Input: part model. Units: mm. Frame: model coordinates. A direction names the side the tool comes from. Coordinates: 2 decimals unless noted, no trailing zeros. Write each loop counter-clockwise with the first axis right and the second up, starting at its lowest first coordinate (ties: lowest second). Pieces come first, ordered by that corner, then holes. Notation, with made-up numbers: M -23,52 L 23,52 A16 ccw 23,72 Z; hole C -28.75,43.5 d3. An arc over 180 degrees is marked long. Use one line per item in the form item = value.
from build123d import *

# Parameters (mm, degrees)
SKETCH1_W                                       = 38.5
SKETCH1_H                                       = 70.536099416
BOSS_EXTRUDE1_DEPTH                             = 38
BOSS_EXTRUDE2_DEPTH                             = 4
BOSS_EXTRUDE3_START                             = -70.536099
BOSS_EXTRUDE3_DEPTH                             = 4
SKETCH4_W                                       = 62.536099416
SKETCH4_H                                       = 60
SKETCH4_R                                       = 17
SKETCH4_R_2                                     = 2.5
BOSS_EXTRUDE4_DEPTH                             = 2
CSK_FOR_M6_FLAT_HEAD_MACHINE_SCREW1_D           = 6.6
CSK_FOR_M6_FLAT_HEAD_MACHINE_SCREW1_CSINK_D     = 12.6
CSK_FOR_M6_FLAT_HEAD_MACHINE_SCREW1_CSINK_ANGLE = 90


with BuildPart() as part:
    # Sketch1 → Boss-Extrude1 (new body)
    with BuildSketch(Plane(origin=(0, 0, 502.500831462), x_dir=(1, 0, 0), z_dir=(0, 0, -1))):
        with Locations((165.241839146, 0)):
            Rectangle(SKETCH1_W, SKETCH1_H)
    extrude(amount=BOSS_EXTRUDE1_DEPTH)

    # Sketch3 → Boss-Extrude2 (add)
    with BuildSketch(Plane(origin=(0, 35.268049708, 0), x_dir=(-1, 0, 0), z_dir=(0, 1, 0))):
        Polygon((-184.491839146, 404.500831462), (-179.491839146, 404.500831462), (-145.991839146, 464.500831462), (-184.491839146, 464.500831462), align=None)
    extrude(amount=-BOSS_EXTRUDE2_DEPTH)

    # Sketch3<2> → Boss-Extrude3 (add)
    with BuildSketch(Plane(origin=(0, 35.268049708, 0), x_dir=(-1, 0, 0), z_dir=(0, 1, 0)).offset(BOSS_EXTRUDE3_START)):
        Polygon((-184.491839146, 404.500831462), (-179.491839146, 404.500831462), (-145.991839146, 464.500831462), (-184.491839146, 464.500831462), align=None)
    extrude(amount=BOSS_EXTRUDE3_DEPTH)

    # Sketch4 → Boss-Extrude4 (add)
    with BuildSketch(Plane.YZ.offset(184.491839146)):
        with Locations((0, 434.500831462)):
            Rectangle(SKETCH4_W, SKETCH4_H)
        with Locations(Location((0, 424.500831462, 0), (0, 0, 270))):
            Circle(SKETCH4_R, mode=Mode.SUBTRACT)
        with Locations(Location((-24.75, 459.250831462, 0), (0, 0, 270))):
            Circle(SKETCH4_R_2, mode=Mode.SUBTRACT)
        with Locations(Location((24.75, 459.250831462, 0), (0, 0, 270))):
            Circle(SKETCH4_R_2, mode=Mode.SUBTRACT)
        with Locations(Location((24.75, 409.750831462, 0), (0, 0, 270))):
            Circle(SKETCH4_R_2, mode=Mode.SUBTRACT)
        with Locations(Location((-24.75, 409.750831462, 0), (0, 0, 270))):
            Circle(SKETCH4_R_2, mode=Mode.SUBTRACT)
    extrude(amount=-BOSS_EXTRUDE4_DEPTH)

    # CSK for M6 Flat Head Machine Screw1 (through all)
    with Locations(Plane(origin=(0, 0, 464.500831462), x_dir=(1, 0, 0), z_dir=(0, 0, -1))):
        with Locations((160.991839146, -18.731950292), (160.991839146, 21.268049708)):
            CounterSinkHole(CSK_FOR_M6_FLAT_HEAD_MACHINE_SCREW1_D / 2, CSK_FOR_M6_FLAT_HEAD_MACHINE_SCREW1_CSINK_D / 2, counter_sink_angle=CSK_FOR_M6_FLAT_HEAD_MACHINE_SCREW1_CSINK_ANGLE)


solid = part.part
(1) First-contact query: pin 1 Ø4 at (y, z) = (-24.75, 409.75) entering from -X; pin 2 Ø3 at (x, y) = (160, 13) entering from -Z. Flat tips, straight axial feed; report the tip coordinate or a pass-through.
Computed:
pin_1 = through
pin_2 = 464.5
(2) Section query A-A on y = 0. Return the cut outline in (x, z).
Computed:
outline = M 145.99,464.5 L 182.49,464.5 L 182.49,441.5 L 184.49,441.5 L 184.49,502.5 L 145.99,502.5 Z; M 182.49,404.5 L 184.49,404.5 L 184.49,407.5 L 182.49,407.5 Z
(3) Section query C-C on x = 153. Return the cut outline in (y, z).
Computed:
outline = M -35.27,451.95 L -31.27,451.95 L -31.27,464.5 L 31.27,464.5 L 31.27,451.95 L 35.27,451.95 L 35.27,502.5 L -35.27,502.5 Z
(4) Pull-direction query (Y, two-part tool) for faces 3 (the flat face through (183, 0, 404.501)), 4 (the cylindrical face through (157.943, -20.004, 485.246)), 5 (the flat face through (170, 35.268, 465)), 6 (the flat face through (169, 31.268, 442)); classes: pulls with the +Y half, pulls with the -Y half, needs draft (parallel to the pull), parting line crosses it, or undercut.
Computed:
face_3 = needs draft
face_4 = undercut
face_5 = pulls with the +Y half
face_6 = undercut
(5) Line query: probe 1 along Y at (x, z) = (180.5, 415); probe 2 along Y at (x, z) = (164, 467); probe 3 along Z at (x, y) = (155, 7). Output: solid intervals per line, ascending.
Computed:
probe_1 = -35.27 to -31.27, 31.27 to 35.27
probe_2 = -35.27 to -23.59, -18.94 to 16.41, 21.06 to 35.27
probe_3 = 464.5 to 502.5
(6) Set-up query: faces 1 (the flat face through (169, -31.268, 442)), 2 (the flat face through (184.492, 0, 465)). Return all of +Z, -Z, +X, -X, +Y, -Y with unobstructed straight access to the full face (end or side cutting, diameter ignored); none if empty.
Computed:
face_1 = -Z, -X
face_2 = +Z, -Z, +X, +Y, -Y
(7) Section query D-D on z = 450.5. Return the cut outline in (x, y), plus the area to 3 significant figures.
Computed:
outline = M 153.81,-35.27 L 184.49,-35.27 L 184.49,35.27 L 153.81,35.27 L 153.81,31.27 L 182.49,31.27 L 182.49,-31.27 L 153.81,-31.27 Z
area = 371 mm^2
(8) Section query B-B on z = 435. Return the cut outline in (x, y), plus the area to 3 significant figures.
Computed:
outline = M 162.46,-35.27 L 184.49,-35.27 L 184.49,-13.37 L 182.49,-13.37 L 182.49,-31.27 L 162.46,-31.27 Z; M 162.46,31.27 L 182.49,31.27 L 182.49,13.37 L 184.49,13.37 L 184.49,35.27 L 162.46,35.27 Z
area = 248 mm^2
